Read the model definition and answer for the solid it produces. Units are mm, in the model's axes. Coordinates: 2 decimals unless noted, no trailing zeros. Write each loop counter-clockwise with the first axis right and the second up, starting at its lowest first coordinate (ties: lowest second). Pieces come first, ordered by that corner, then holes. Notation, with made-up numbers: (18, 74) -> (27, 74) arc R9 cw to (27, 84) -> close; hole circle Ø10 at (-37.75, 50.25). An arc over 180 degrees is marked (long way). One line per item, written item: value. Start each with the question number.
1. For a pull along Z with two mould halves and no side action, classify faces 1 (the flat face through (-78.595, -100, -17)), 2 (the cylindrical face through (-7.98, -100.18, -100.42)), 3 (the flat face through (-69, -100, 98.976)) as pulls with the +Z half, pulls with the -Z half, needs draft (parallel to the pull), parting line crosses it, or undercut.
2. Find section B-B, the plane y = -94. Write down the section's boundary in (x, z), and give its area (3 significant figures).
3. Find section C-C, the plane z = -23. Write down the section's boundary in (x, y), and give its area (3 significant figures).
4. Find section A-A, the plane x = -8.5. Write down the section's boundary in (y, z), and give its area (3 significant figures).
5. Consider line 1 along Z through (x, y) = (-73, -140.5); line 2 along Z through (x, y) = (-67, -101); line 3 along Z through (x, y) = (-4.5, -59). Determine where each line is inside the solid, lowest interval first.
6. Find section D-D, the plane x = -38.5. Write down the section's boundary in (y, z).
7. Given P1, Ø3, axis at x = -66, y = -167, coming from the -Z side; P2, Ø6, axis at y = -129.5, z = -25, coming from the +X side; P3, Ø4, axis at x = -33, y = -67, coming from the +Z side, each flat-ended and moving along its own axis, determine where each tip first touches the part or whether it passes through.
```python
from build123d import *

# Parameters (mm, degrees)
F1_DEPTH = 203.2


with BuildPart() as f1:
    # F0 (on Front) → F1 (new body)
    with BuildSketch(Plane.XZ):
        with BuildLine():
            Line((-60.342863, 98.975755), (-78.595482, 98.975755))
            Line((-78.595482, 98.975755), (-78.595482, -137.244245))
            ThreePointArc((-78.595482, -137.244245), (-7.380595, -99.388032), (-11.104383, -18.822614))
            ThreePointArc((-11.104383, -18.822614), (-16.753261, 11.099402), (0.737776, 36.025302))
            ThreePointArc((0.737776, 36.025302), (-16.486267, 80.421272), (-60.342863, 98.975755))
        make_face()
    extrude(amount=F1_DEPTH)


solid = f1.part
```
Answer block:
1. face 1: needs draft
1. face 2: undercut
1. face 3: pulls with the +Z half
2. outline: (-78.6, -137.24) arc R75.41 ccw to (-11.1, -18.82) arc R39.17 cw to (0.74, 36.03) arc R61.11 ccw to (-60.34, 98.98) -> (-78.6, 98.98) -> close
2. area: 16,000 mm2
3. outline: (-78.6, -203.2) -> (-8.38, -203.2) -> (-8.38, 0) -> (-78.6, 0) -> close
3. area: 14,300 mm2
4. outline: (-203.2, -101.29) -> (0, -101.29) -> (0, -22.81) -> (-203.2, -22.81) -> close; (-203.2, 27.98) -> (0, 27.98) -> (0, 70.22) -> (-203.2, 70.22) -> close
4. area: 24,500 mm2
5. line 1: z = -137.46 to 98.98
5. line 2: z = -137.23 to 98.98
5. line 3: z = -93.81 to -30.29, 32.1 to 62.68
6. outline: (-203.2, -129.16) -> (0, -129.16) -> (0, 94.94) -> (-203.2, 94.94) -> close
7. P1: stops at z = -137.27
7. P2: stops at x = -5.61
7. P3: stops at z = 93.47
